Study the drawing (mm; zero at the part's minimum x, y, z) and answer. A direction names the side the tool comes from. Coordinates: 2 decimals unless noted, no trailing zeros. Loops run counter-clockwise (first coordinate to the right, second up) from the corner with the lowest first, then second, coordinate; pieces in that order, holes last. Notation, with made-up numbers: (-32.5, 48) -> (-26.5, 48) arc R12 ccw to (-26.5, 70) -> close; hole circle Ø5 at (33, 73). An arc over 180 degrees is marked (long way). Answer in a Markdown table with one row per item.
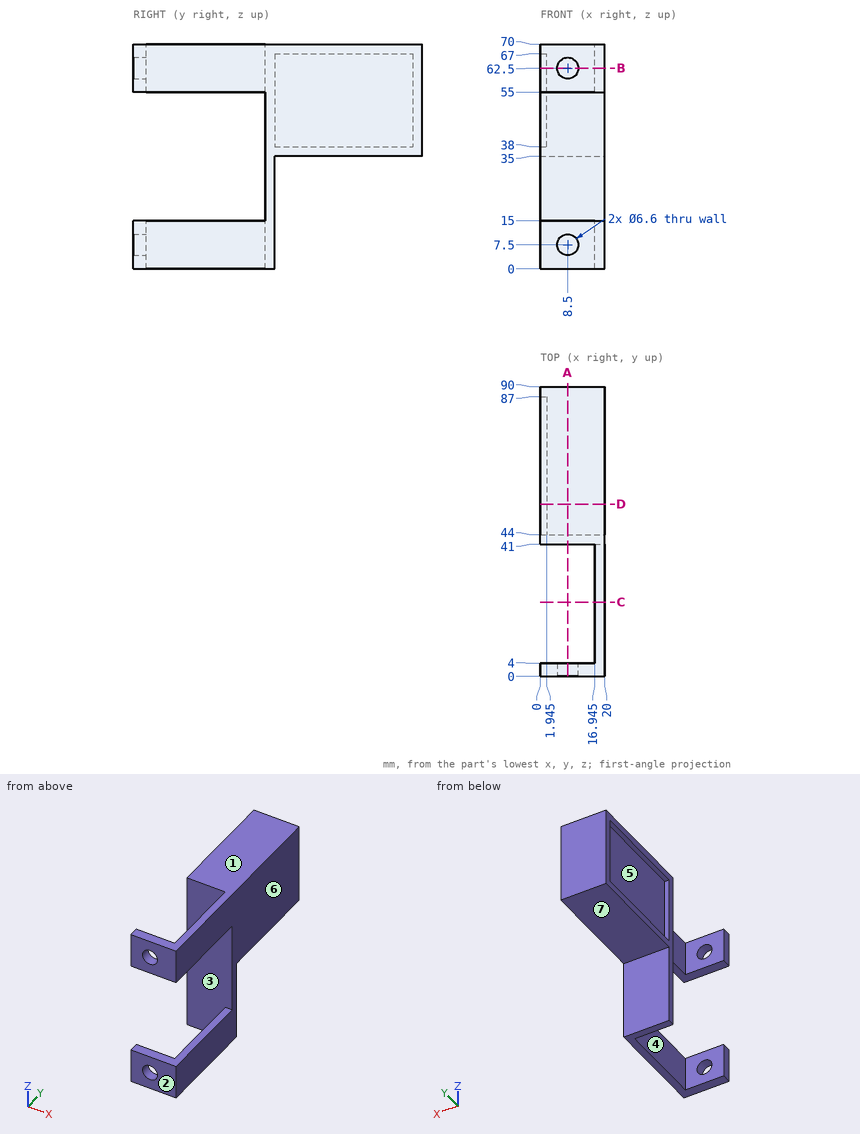
1. The mould has two halves that part along Y. Classify the marked faces 1, 2 and 3: pulls with the +Y half, pulls with the -Y half, needs draft (parallel to the pull), parting line crosses it, or undercut.
A:
| item | result |
|---|---|
| face 1 | needs draft |
| face 2 | pulls with the -Y half |
| face 3 | undercut |
2. A cutting plane is placed at C-C on y = 23. Give the vertices of the cut face in (x, z) (3 decimals).
A:
| item | result |
|---|---|
| outline | (16.945, 0) -> (20, 0) -> (20, 15) -> (16.945, 15) -> close; (16.945, 55) -> (20, 55) -> (20, 70) -> (16.945, 70) -> close |
3. Find the intervals of material crossed by probe 1 along Z at (x, y) = (8.5, 1.55); probe 2 along Y at (x, z) = (15.5, 24); probe 3 along Z at (x, y) = (8.25, 81.5), in increasing order.
A:
| item | result |
|---|---|
| probe 1 | z = 0 to 4.2, 10.8 to 15, 55 to 59.2, 65.8 to 70 |
| probe 2 | y = 41 to 44 |
| probe 3 | z = 35 to 70 |
4. A tool of negligible diameter and unlimited length cuts with its end or side. For the marked faces 4, 5, 6 and 7, from which of +Z, -Z, +X, -X, +Y, -Y can it reach the whole face along a straight path? Write none if from no direction.
A:
| item | result |
|---|---|
| face 4 | +Z, -Z, -X |
| face 5 | -X |
| face 6 | +Z, -Z, +X, +Y, -Y |
| face 7 | -Z, +X, -X, +Y |
5. A cutting plane is placed at B-B on z = 62.5. Give the vertices of the cut face in (x, y) (3 decimals).
A:
| item | result |
|---|---|
| outline | (0, 0) -> (5.2, 0) -> (5.2, 4) -> (0, 4) -> close; (0, 41) -> (16.945, 41) -> (16.945, 4) -> (11.8, 4) -> (11.8, 0) -> (20, 0) -> (20, 90) -> (0, 90) -> (0, 87) -> (1.945, 87) -> (1.945, 44) -> (0, 44) -> close |
6. A cutting plane is placed at A-A on x = 8.5. Give the vertices of the cut face in (y, z).
A:
| item | result |
|---|---|
| outline | (0, 0) -> (4, 0) -> (4, 4.2) -> (0, 4.2) -> close; (0, 10.8) -> (4, 10.8) -> (4, 15) -> (0, 15) -> close; (0, 55) -> (4, 55) -> (4, 59.2) -> (0, 59.2) -> close; (0, 65.8) -> (4, 65.8) -> (4, 70) -> (0, 70) -> close; (41, 0) -> (44, 0) -> (44, 35) -> (90, 35) -> (90, 70) -> (41, 70) -> close |
7. A cutting plane is placed at D-D on y = 53.5. Give the vertices of the cut face in (x, z) (3 decimals), and give its area (3 significant figures).
A:
| item | result |
|---|---|
| outline | (0, 35) -> (20, 35) -> (20, 70) -> (0, 70) -> (0, 67) -> (1.945, 67) -> (1.945, 38) -> (0, 38) -> close |
| area | 644 mm2 |
8. Given pin 1 Ø8.5 at (y, z) = (70.5, 53.5) entering from -X (3 decimals); pin 2 Ø5 at (x, z) = (15.5, 10) entering from +Y; pin 3 Ø5 at (x, z) = (11, 18) entering from -Y, each flat-ended and moving along its own axis, determine where each tip first touches the part or whether it passes through.
A:
| item | result |
|---|---|
| pin 1 | stops at x = 1.945 |
| pin 2 | stops at y = 44 |
| pin 3 | stops at y = 41 |
